Input: part model. Units: mm. Frame: model coordinates. A direction names the side the tool comes from. Give positions to 0.01 mm unless a question says otherwise; leave off trailing zeros. Write each loop counter-clockwise with the first axis right and the second up, starting at its lowest first coordinate (ties: lowest second). Pieces come first, ordered by that corner, then holes. Notation, with made-up numbers: (74, -15) - (83, -15) arc R7 cw to (83, -3) - close; hole circle Ø9 at (-35, 61.25). An arc over 180 degrees is marked (long way). Answer as CSV lines item,"result". Start each with the question number.
Autodesk Inventor part; units mm, degrees
ref_plane "YZ Plane" through (0, 0, 0) normal (1, 0, 0) x (0, 1, 0)
ref_plane "XZ Plane" through (0, 0, 0) normal (0, 1, 0) x (-1, 0, 0)
ref_plane "XY Plane" through (0, 0, 0) normal (0, 0, 1) x (1, 0, 0)
sketch "Sketch1" plane through (0, 0, 0) normal (0, 1, 0) x (-1, 0, 0)
  circle A0 centre (0, 0) radius 2
  circle A1 centre (0, 0) radius 1.75
  dimension "d0" = 4
  dimension "d3" = 3.5
extrude "Beams" add sketch "Sketch1" along normal blind 30 contours A0 | A1
sketch "Sketch3" plane through (0, 0, 0) normal (0, -1, 0) x (1, 0, 0)
  circle A0 centre (0, 0) radius 1.5
  dimension "d4" = 3
extrude "Screw Hole" cut sketch "Sketch3" against normal blind 10
thread "Thread1"
sketch "Sketch4" plane through (0, 30, 0) normal (0, 1, 0) x (1, 0, 0)
  circle A0 centre (0, 0) radius 1.5
  dimension "d9" = 3
extrude "Extrusion3" cut sketch "Sketch4" against normal blind 10
thread "Thread2"
properties part number "Beams"
1) Reachability of faces 4 (the cylindrical face through (-1.5, 25.07, -0.07)), 5 (the flat face through (0, 10, 0)) from +Z, -Z, +X, -X, +Y, -Y: full face, straight path, thin tool, end or side. Return the list, or none.
2) Cut plane B-B on z = 1.1. Output: boundary loops of the cut face in (x, y), and give its area (3 significant figures).
3) Cut plane A-A on x = 0. Output: boundary loops of the cut face in (y, z).
4) Cut plane C-C on y = 9.5. Output: boundary loops of the cut face in (x, z).
5) Material intervals for line 1 (Z direction, x = 0, y = 5); line 2 (Y direction, x = -0.3, z = -0.55); line 3 (X direction, y = 7, z = 1), sorted ascending. Write a range as from..to.
6) Pull-direction query (Z, two-part tool) for faces 1 (the flat face through (0, 20, 0)), 2 (the cylindrical face through (-1.5, 4.93, 0.07)), 3 (the cylindrical face through (0, 15, 2)); classes: +Z half, -Z half, draft (parallel to the pull), parting line (faces both ways), or undercut.
7) Cut plane D-D on y = 17.5. Output: boundary loops of the cut face in (x, z).
8) Contact query for flat-ended pins moving along their axis: P1, Ø1.8, axis at x = 0, z = 0, coming from the -Y side; P2, Ø1, axis at x = -1, y = 24, coming from the +Z side. Output: stop coordinate, or through.
Numbers:
1,face 4,"+Y"
1,face 5,"-Y"
2,outline,"(-1.67, 0) - (-1.02, 0) - (-1.02, 10) - (1.02, 10) - (1.02, 0) - (1.67, 0) - (1.67, 30) - (1.02, 30) - (1.02, 20) - (-1.02, 20) - (-1.02, 30) - (-1.67, 30) - close"
2,area,"59.4 mm²"
3,outline,"(0, -2) - (30, -2) - (30, -1.5) - (20, -1.5) - (20, 1.5) - (30, 1.5) - (30, 2) - (0, 2) - (0, 1.5) - (10, 1.5) - (10, -1.5) - (0, -1.5) - close"
4,outline,"circle Ø4 at (0, 0); hole circle Ø3 at (0, 0)"
5,line 1,"z = -2..-1.5, 1.5..2"
5,line 2,"y = 10..20"
5,line 3,"x = -1.73..-1.12, 1.12..1.73"
6,face 1,"undercut"
6,face 2,"undercut"
6,face 3,"parting line"
7,outline,"circle Ø4 at (0, 0)"
8,P1,"stops at y = 10"
8,P2,"stops at z = 1.94"
